Verification items for the finished model (mm, model axes). Face numbers are marked on the shaded views. Coordinates: 2 decimals unless noted, no trailing zeros. Write each loop counter-clockwise with the first axis right and the second up, starting at its lowest first coordinate (ties: lowest second). Pieces come first, ordered by that corner, then holes. Notation, with made-up numbers: (-32.75, -35.5) - (18.25, -35.5) arc R29 cw to (18.25, -4.5) - close; hole circle Ø4 at (18.5, 32). An arc over 180 degrees is marked (long way). Answer as CSV lines item,"result". Start each with the question number.
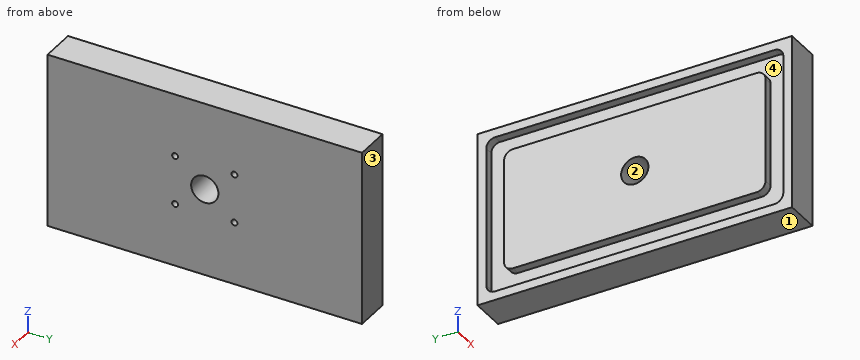
Autodesk Inventor part; units mm, degrees
ref_plane "YZ Plane" through (0, 0, 0) normal (1, 0, 0) x (0, 1, 0)
ref_plane "XZ Plane" through (0, 0, 0) normal (0, 1, 0) x (-1, 0, 0)
ref_plane "XY Plane" through (0, 0, 0) normal (0, 0, 1) x (1, 0, 0)
sketch "Sketch1" plane through (0, 0, 0) normal (1, 0, 0) x (0, 1, 0)
  line L0 (57.15, 31.75) -> (-57.15, 31.75)
  line L1 (-57.15, 31.75) -> (-57.15, -31.75)
  line L2 (-57.15, -31.75) -> (57.15, -31.75)
  line L3 (57.15, -31.75) -> (57.15, 31.75)
  line L4 (-50.8, 25.4) -> (50.8, 25.4)
  line L5 (50.8, 25.4) -> (50.8, -25.4)
  line L6 (50.8, -25.4) -> (-50.8, -25.4)
  line L7 (-50.8, -25.4) -> (-50.8, 25.4)
  point P0 (0, 0)
  point P1 (0, -31.75)
  point P2 (57.15, 0)
  point P3 (0, 25.4)
  point P4 (-50.8, 0)
  dimension "d0" = 63.5
  dimension "d1" = 114.3
  dimension "d14" = 50.8
  dimension "d15" = 101.6
extrude "Extrusion1" add sketch "Sketch1" along normal blind 12.7 contours L3 L2 L1 L0 | L4 L5 L6 L7
sketch "Sketch2" plane through (12.7, 0, 0) normal (1, 0, 0) x (0, 0, -1)
  line L0 (-8.89, -10.795) -> (8.89, 10.795) construction
  line L1 (-8.89, 10.795) -> (8.89, -10.795) construction
  circle A0 centre (0, 0) radius 4.9609
  dimension "d5" = 21.59
  dimension "d12" = 9.9219
  dimension "d13" = 17.78
sketch "Sketch3" plane through (0, 0, 0) normal (-1, 0, 0) x (0, 0, 1)
  line L0 (-28.575, -53.975) -> (28.575, -53.975)
  line L1 (28.575, -53.975) -> (28.575, 53.975)
  line L2 (28.575, 53.975) -> (-28.575, 53.975)
  line L3 (-28.575, 53.975) -> (-28.575, -53.975)
  line L4 (22.098, 47.498) -> (22.098, -47.498)
  line L5 (22.098, -47.498) -> (-22.098, -47.498)
  line L6 (-22.098, -47.498) -> (-22.098, 47.498)
  line L7 (-22.098, 47.498) -> (22.098, 47.498)
  point P0 (0, 0)
  point P1 (0, -53.975)
  point P2 (-28.575, 0)
  point P3 (0, 0)
  point P4 (28.575, 0)
  point P5 (0, 53.975)
  dimension "d16" = 107.95
  dimension "d17" = 57.15
  dimension "d31" = 6.477
extrude "Extrusion3" cut sketch "Sketch3" against normal blind 3.175
extrude "Extrusion4" cut sketch "Sketch2" against normal through all
hole "Hole1" at (12.7, -10.795, 8.89) at (12.7, 10.795, 8.89) at (12.7, 10.795, -8.89) at (12.7, -10.795, -8.89) direction (-1, 0, 0) diameter 2.159 depth 8.8646 tip angle 118
fillet "Fillet1" radius 3.175 8 edges at (1.5875, 53.975, 28.575) (1.5875, -47.498, 22.098) (1.5875, -47.498, -22.098) (1.5875, -53.975, -28.575) (1.5875, 47.498, -22.098) (1.5875, -53.975, 28.575) (1.5875, 53.975, -28.575) (1.5875, 47.498, 22.098)
properties part number "plate" material "Aluminum 6061"
1. Scan lines: line 1 along Y through (x, z) = (7.25, 8.89); line 2 along Y through (x, z) = (3, 6) (3 decimals); line 3 along Z through (x, y) = (0.75, 38.5) (3 decimals). Record each from-to range of solid material in increasing order. Write a range as from..to.
2. Cross-section at D-D (y = -23). Record the cut outline in (x, z) (3 decimals), and give its area (3 significant figures).
3. Draft check along Z on the marked faces 1, 2, 3 and 4. Enter one of: pulls with the +Z half, pulls with the -Z half, needs draft (parallel to the pull), parting line crosses it, or undercut.
4. Cross-section at A-A (y = 0). Record the cut outline in (x, z) (3 decimals).
5. Cross-section at C-C (z = -16.5). Record the cut outline in (x, y) (3 decimals), and give its area (3 significant figures).
6. Cross-section at B-B (z = 0). Record the cut outline in (x, y) (3 decimals).
Completed:
1,line 1,"y = -57.15..-11.87, -9.72..9.72, 11.87..57.15"
1,line 2,"y = -57.15..-53.975, -47.498..47.498, 53.975..57.15"
1,line 3,"z = -31.75..-28.575, -22.098..22.098, 28.575..31.75"
2,outline,"(0, -31.75) - (12.7, -31.75) - (12.7, 31.75) - (0, 31.75) - (0, 28.575) - (3.175, 28.575) - (3.175, 22.098) - (0, 22.098) - (0, -22.098) - (3.175, -22.098) - (3.175, -28.575) - (0, -28.575) - close"
2,area,"765 mm2"
3,face 1,"pulls with the -Z half"
3,face 2,"undercut"
3,face 3,"needs draft"
3,face 4,"undercut"
4,outline,"(0, -31.75) - (12.7, -31.75) - (12.7, -4.961) - (0, -4.961) - (0, -22.098) - (3.175, -22.098) - (3.175, -28.575) - (0, -28.575) - close; (0, 4.961) - (12.7, 4.961) - (12.7, 31.75) - (0, 31.75) - (0, 28.575) - (3.175, 28.575) - (3.175, 22.098) - (0, 22.098) - close"
5,outline,"(0, -57.15) - (12.7, -57.15) - (12.7, 57.15) - (0, 57.15) - (0, 53.975) - (3.175, 53.975) - (3.175, 47.498) - (0, 47.498) - (0, -47.498) - (3.175, -47.498) - (3.175, -53.975) - (0, -53.975) - close"
5,area,"1,410 mm2"
6,outline,"(0, -57.15) - (12.7, -57.15) - (12.7, -4.961) - (0, -4.961) - (0, -47.498) - (3.175, -47.498) - (3.175, -53.975) - (0, -53.975) - close; (0, 4.961) - (12.7, 4.961) - (12.7, 57.15) - (0, 57.15) - (0, 53.975) - (3.175, 53.975) - (3.175, 47.498) - (0, 47.498) - close"
